from build123d import *

# Parameters (mm, degrees)
BOSS_EXTRUDE1_DEPTH     = 101.6
SKETCH5_R               = 5.08
CUT_EXTRUDE4_DEPTH      = 168.213364787
CUT_EXTRUDE5_DEPTH      = 168.213364787
CUT_EXTRUDE5_DEPTH_BACK = 168.213364787
FILLET1_R               = 2.54


with BuildPart() as part:
    # Sketch1 → Boss-Extrude1 (new body)
    with BuildSketch(Plane(origin=(0, 0, 0), x_dir=(0, 0, -1), z_dir=(1, 0, 0))):
        with BuildLine():
            Line((11.639742265, -5.08), (113.239742265, -5.08))
            Line((113.239742265, -5.08), (132.198560368, 0))
            Line((132.198560368, 0), (113.239742265, 5.08))
            Line((113.239742265, 5.08), (11.639742265, 5.08))
            ThreePointArc((11.639742265, 5.08), (-12.7, 0), (11.639742265, -5.08))
        make_face()
    extrude(amount=BOSS_EXTRUDE1_DEPTH)

    # Sketch5 → Cut-Extrude4 (cut, through all)
    with BuildSketch(Plane(origin=(101.6, 0, 0), x_dir=(0, 0, -1), z_dir=(1, 0, 0))):
        Circle(SKETCH5_R)
    extrude(amount=-CUT_EXTRUDE4_DEPTH, mode=Mode.SUBTRACT)

    # Sketch6 → Cut-Extrude5 (cut, two sides: drawn at the far end of the back side and taken through both)
    with BuildSketch(Plane(origin=(0, 0, 0), x_dir=(1, 0, 0), z_dir=(0, 1, 0)).offset(-CUT_EXTRUDE5_DEPTH_BACK)):
        Polygon((0, 132.198560368), (0, 113.239742265), (18.958818102, 132.198560368), align=None)
        Polygon((101.6, 132.198560368), (101.6, 113.239742265), (82.641181898, 132.198560368), align=None)
    extrude(amount=CUT_EXTRUDE5_DEPTH + CUT_EXTRUDE5_DEPTH_BACK, mode=Mode.SUBTRACT)

    # Fillet1
    fillet1_edges = [part.edges().sort_by_distance(p)[0] for p in [
        (50.8, 5.08, -11.639742265),
        (50.8, -5.08, -11.639742265),
    ]]
    fillet(fillet1_edges, radius=FILLET1_R)


solid = part.part
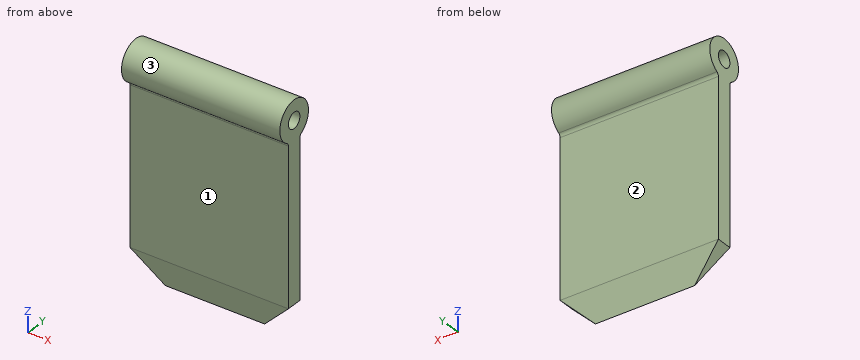
Input: part model. Units: mm. Frame: model coordinates. Face numbers are marked on the shaded views. A direction names the side the tool comes from. Coordinates: 2 decimals unless noted, no trailing zeros. Loops run counter-clockwise (first coordinate to the right, second up) from the corner with the lowest first, then second, coordinate; pieces in that order, holes last. Notation, with made-up numbers: (71.25, 26) -> (106.25, 26) arc R10 ccw to (106.25, 35) -> close; hole circle Ø9 at (27, -38). An arc over 180 degrees is marked (long way). Write each question's results on one line, items separated by ' | '. Start each with the question number.
Q1. Pin query (flat end, axial travel): pin 1 (1.5 mm diameter, centred on x = 38.5, z = -77, fed in from +Y); pin 2 (5 mm diameter, centred on x = 72, z = -110.5, fed in from -Y); pin 3 (3 mm diameter, centred on y = -2.5, z = -116.5, fed in from -X). Return the tip coordinate at first contact, or that it passes through.
Q2. Reachability of the marked faces 1, 2 and 3 from +Z, -Z, +X, -X, +Y, -Y: full face, straight path, thin tool, end or side. Return the list, or none.
Q3. Section A-A, the plane z = 0. Return the cut outline in (x, y).
Q4. Section D-D, the plane z = -18. Return the cut outline in (x, y).
Q5. Ray query, line 1 (Y direction, x = 59.5, z = -42); line 2 (Z direction, x = 38.5, y = -8); line 3 (X direction, y = 0.75, z = -117). Return the intervals inside material, ascending. Write a range as from..to.
Q6. Section C-C, the plane y = -2. Return the cut outline in (x, z), plus the area to 3 significant figures.
Q7. Section B-B, the plane x = 24. Return the cut outline in (y, z).
Found:
1) pin 1: y = 5.08 | pin 2: y = -5.08 | pin 3: x = 1.76
2) face 1: -Z, +X, -X, -Y | face 2: -Z, +X, -X, +Y | face 3: +X, -X
3) outline: (0, -12.7) -> (101.6, -12.7) -> (101.6, -5.08) -> (0, -5.08) -> close; (0, 5.08) -> (101.6, 5.08) -> (101.6, 12.7) -> (0, 12.7) -> close
4) outline: (0, -5.08) -> (101.6, -5.08) -> (101.6, 5.08) -> (0, 5.08) -> close
5) line 1: -5.08..5.08 | line 2: -9.86..9.86 | line 3: 3.76..97.84
6) outline: (0, -113.24) -> (11.49, -124.73) -> (90.11, -124.73) -> (101.6, -113.24) -> (101.6, -4.67) -> (0, -4.67) -> close; (0, 4.67) -> (101.6, 4.67) -> (101.6, 12.54) -> (0, 12.54) -> close | area: 12,900 mm2
7) outline: (-6.35, -11) arc R2.54 cw to (-5.08, -13.2) -> (-5.08, -113.24) -> (0, -132.2) -> (5.08, -113.24) -> (5.08, -13.2) arc R2.54 cw to (6.35, -11) arc R12.7 ccw (long way) to start; hole circle Ø10.16 at (0, 0)
